```python
from build123d import *

# Parameters (mm, degrees)
ESQUISSE1_R             = 25
ESQUISSE1_R_2           = 1.7
BOSS_EXTRU_1_DEPTH      = 5
ESQUISSE11_R            = 0.8
ENL_V_MAT_EXTRU_1_DEPTH = 36.707142143
ESQUISSE13_W            = 4.903660669
ESQUISSE13_H            = 28.894120166
ENL_V_MAT_EXTRU_2_DEPTH = 36.707142143


with BuildPart() as part:
    # Esquisse1 → Boss.-Extru.1 (new body)
    with BuildSketch(Plane.XY):
        Circle(ESQUISSE1_R)
        with Locations((-13.435028843, 13.435028843)):
            Circle(ESQUISSE1_R_2, mode=Mode.SUBTRACT)
        with Locations((13.435028843, 13.435028843)):
            Circle(ESQUISSE1_R_2, mode=Mode.SUBTRACT)
        with Locations((13.435028843, -13.435028843)):
            Circle(ESQUISSE1_R_2, mode=Mode.SUBTRACT)
        with Locations((-13.435028843, -13.435028843)):
            Circle(ESQUISSE1_R_2, mode=Mode.SUBTRACT)
    extrude(amount=BOSS_EXTRU_1_DEPTH)

    # Esquisse11 → Enlèv. mat.-Extru.1 (cut, through all)
    with BuildSketch(Plane(origin=(0, 0, 0), x_dir=(-1, 0, 0), z_dir=(0, 0, -1))):
        with Locations((0, 7.398882196)):
            Circle(ESQUISSE11_R)
        with Locations((5.827506735, 5.634287936)):
            Circle(ESQUISSE11_R)
        with Locations((5.827506735, -5.758693792)):
            Circle(ESQUISSE11_R)
        with Locations((0, -7.398882196)):
            Circle(ESQUISSE11_R)
        with Locations((-5.645080413, -5.758693792)):
            Circle(ESQUISSE11_R)
        with Locations((-5.645080413, 5.634287936)):
            Circle(ESQUISSE11_R)
    extrude(amount=-ENL_V_MAT_EXTRU_1_DEPTH, mode=Mode.SUBTRACT)

    # Esquisse13 → Enlèv. mat.-Extru.2 (cut, through all)
    with BuildSketch(Plane(origin=(0, 0, 0), x_dir=(-1, 0, 0), z_dir=(0, 0, -1))):
        with Locations((23.534998976, -1.01203124)):
            Rectangle(ESQUISSE13_W, ESQUISSE13_H)
    extrude(amount=-ENL_V_MAT_EXTRU_2_DEPTH, mode=Mode.SUBTRACT)


solid = part.part
```
The model under review builds one solid part; all positions refer to its coordinate system, in mm. Give positions to 0.01 mm unless a question says otherwise; leave off trailing zeros. Order: outer loops, then holes, each group sorted by start corner. A loop starts at its lowest first (then second) coordinate and runs counter-clockwise, first axis right, second up. Notation, with made-up numbers: (26.25, 44) - (79.25, 44) arc R10 cw to (79.25, 57) - close; hole circle Ø6 at (-37, 39.25). An arc over 180 degrees is marked (long way). Use CSV: the item, a comma, the result in double quotes. Start each with the question number.
Q1. To check wall thickness, follow line 1 along X through (y, z) = (-5.5, 1.55); line 2 along X through (y, z) = (5, 1.5); line 3 along Y through (x, z) = (-13, 4.55). State the ranges of each line that lie inside material, in increasing order. Write a range as [from, to].
Q2. We need section A-A, the plane x = 0. Write out the cut boundary in (y, z).
Q3. We need section B-B, the plane z = 3.5. State how many separate pieces and enclosed holes the cut face has, and give its area (3 significant figures).
Q4. The part is to be moulded in two halves that separate along X. For faces 1 (the cylindrical face through (24.984, -0.901, 2.465)), 2 (the cylindrical face through (-14.69, 14.58, 2.46)), 3 (the flat face through (2, 0, 0)), say which applies: +X half, -X half, draft (parallel to the pull), parting line (faces both ways), or undercut.
Q5. We need section C-C, the plane y = 16. Write out the cut boundary in (x, z).
Q6. Clearance check with flat-ended pins moving along their axes: pin 1 Ø1.4 at (x, y) = (0, -7.4) entering from +Z; pin 2 Ø1.5 at (x, z) = (-13, 2) entering from -Y. State where each tip first meets the part, or that it passes through.
Q7. We need section D-D, the plane x = 22.5. Write out the cut boundary in (y, z), and give its area (3 significant figures).
Outcome:
1,line 1,"x = [-21.08, -6.58], [-5.07, 4.89], [6.4, 24.39]"
1,line 2,"x = [-21.08, -6.32], [-5.34, 5.16], [6.13, 24.49]"
1,line 3,"y = [-21.35, -15.08], [-11.79, 11.79], [15.08, 21.35]"
2,outline,"(-25, 0) - (-8.2, 0) - (-8.2, 5) - (-25, 5) - close; (-6.6, 0) - (6.6, 0) - (6.6, 5) - (-6.6, 5) - close; (8.2, 0) - (25, 0) - (25, 5) - (8.2, 5) - close"
3,separate pieces,"1"
3,enclosed holes,"10"
3,area,"1,840 mm^2"
4,face 1,"parting line"
4,face 2,"undercut"
4,face 3,"draft"
5,outline,"(-19.21, 0) - (19.21, 0) - (19.21, 5) - (-19.21, 5) - close"
6,pin 1,"passes through"
6,pin 2,"stops at y = -21.79"
7,outline,"(-10.9, 0) - (10.9, 0) - (10.9, 5) - (-10.9, 5) - close"
7,area,"109 mm^2"
